```python
from build123d import *

# Parameters (mm, degrees)
SKETCH2_R           = 20
SKETCH4_R           = 20
BOSS_EXTRUDE1_DEPTH = 553.90605298
SKETCH5_R           = 20
BOSS_EXTRUDE2_DEPTH = 622
SKETCH6_R           = 17.5
CUT_EXTRUDE1_DEPTH  = 199
SKETCH7_R           = 17.5
BOSS_EXTRUDE3_DEPTH = 84
SKETCH9_R           = 17.5
BOSS_EXTRUDE4_DEPTH = 84


with BuildPart() as part:
    # Sweep1: sweep along a path in Sketch3
    with BuildLine(Plane(origin=(0, 0, 0), x_dir=(0, 0, -1), z_dir=(1, 0, 0))) as sweep1_path:
        Line((0, 0), (0, 302.819820908))
        ThreePointArc((0, 302.819820908), (15.565663847, 340.398657675), (53.144500614, 355.964321522))
        Line((53.144500614, 355.964321522), (550.094321522, 355.964321522))
        Line((550.094321522, 355.964321522), (550.094321522, 0.094321522))
    # Sketch2 → Sweep1 (sweep)
    with BuildSketch(Plane(origin=(0, 0, 0), x_dir=(1, 0, 0), z_dir=(0, 1, 0))):
        Circle(SKETCH2_R)
    sweep(path=sweep1_path.line, transition=Transition.RIGHT)

    # Sketch4 → Boss-Extrude1 (add)
    with BuildSketch(Plane.XZ):
        with Locations(Location((0, 0, 0), (0, 0, 90))):
            Circle(SKETCH4_R)
    extrude(amount=BOSS_EXTRUDE1_DEPTH)

    # Sketch5 → Boss-Extrude2 (add)
    with BuildSketch(Plane.XY):
        Circle(SKETCH5_R)
    extrude(amount=-BOSS_EXTRUDE2_DEPTH)

    # Sketch6 → Cut-Extrude1 (cut)
    with BuildSketch(Plane(origin=(0, 0, -622), x_dir=(-1, 0, 0), z_dir=(0, 0, -1))):
        Circle(SKETCH6_R)
    extrude(amount=-CUT_EXTRUDE1_DEPTH, mode=Mode.SUBTRACT)

    # Sketch7 → Boss-Extrude3 (add)
    with BuildSketch(Plane.XY):
        with Locations((0, -503.90605298)):
            Circle(SKETCH7_R)
    extrude(amount=-BOSS_EXTRUDE3_DEPTH)

    # Sketch9 → Boss-Extrude4 (add)
    with BuildSketch(Plane(origin=(0, 0, 0), x_dir=(0, 0, -1), z_dir=(1, 0, 0))):
        with Locations((0, -503.90605298)):
            Circle(SKETCH9_R)
    extrude(amount=-BOSS_EXTRUDE4_DEPTH)


solid = part.part
```
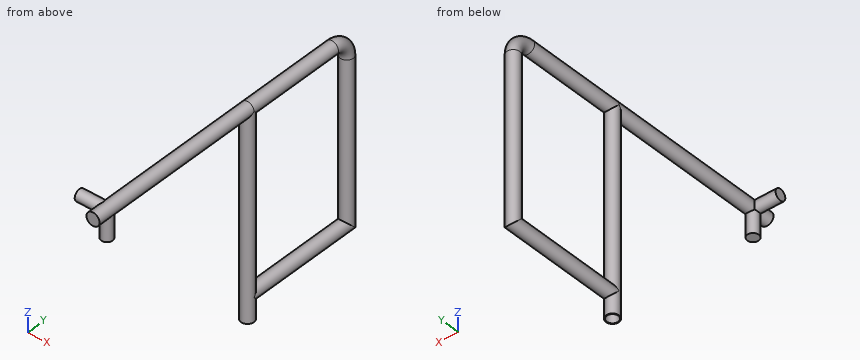
Check sheet for the modelled part. Datum: model origin and axes. Units: mm. Round coordinates to 2 decimals unless told otherwise and drop trailing zeros. Order: outer loops, then holes, each group sorted by start corner. A loop starts at its lowest first (then second) coordinate and runs counter-clockwise, first axis right, second up. Notation, with made-up numbers: (46, 67.25) - (98, 67.25) arc R10 ccw to (98, 77.25) - close; hole circle Ø5 at (46, -29). An arc over 180 degrees is marked (long way). Write item = value, one per line.
Q1. Thickness scan on line 1 along Y through (x, z) = (0, -515); line 2 along Y through (x, z) = (0, -533); line 3 along Z through (x, y) = (3.5, 33). Record the ranges inside material, lowest first.
Computed:
line_1 = -20 to -17.5, 17.5 to 20, 335.96 to 375.96
line_2 = -20 to -17.5, 17.5 to 375.96
line_3 = -569.79 to -530.4, -19.69 to 19.69
Q2. Section check B-B (z = -171). Record the boundary of the cut face in (x, y).
Computed:
outline = circle Ø40 at (0, 0); circle Ø40 at (0, 355.96)
Q3. Section check C-C (y = -142). Record the boundary of the cut face in (x, z), and give its area (3 significant figures).
Computed:
outline = circle Ø40 at (0, 0)
area = 1,260 mm^2
Q4. Section check D-D (x = -51). Record the boundary of the cut face in (y, z).
Computed:
outline = circle Ø35 at (-503.91, 0)
Q5. Section check A-A (x = 0). Record the boundary of the cut face in (y, z), and give its area (3 significant figures).
Computed:
outline = (-553.91, -20) - (-521.41, -20) - (-521.41, -84) - (-486.41, -84) - (-486.41, -20) - (-20, -20) - (-20, -622) - (-17.5, -622) - (-17.5, -423) - (17.5, -423) - (17.5, -622) - (20, -622) - (20, -570.09) - (375.96, -570.09) - (375.96, -53.14) arc R73.14 ccw to (302.82, 20) - (-553.91, 20) - close; hole (20, -530.09) - (335.96, -530.09) - (335.96, -53.14) arc R33.14 ccw to (302.82, -20) - (20, -20) - close
area = 90,300 mm^2
Q6. Go/stop test with a flat-tipped pin: pin 1 (2 mm diameter, centred on x = -3, z = -105.5, fed in from +Y). Record where the tip stops, or that it passes through.
Computed:
pin_1 = 375.86
